Read the model definition and answer for the solid it produces. Units are mm, in the model's axes. A direction names the side the tool comes from. Give positions to 0.01 mm unless a question says otherwise; leave off trailing zeros. Loops run counter-clockwise (first coordinate to the right, second up) from the corner with the lowest first, then second, coordinate; pieces in that order, holes last.
(1) Find section D-D, the plane z = -4.75. Write down the section's boundary in (x, y).
(2) Straight lines are drawn through the part: probe 1 along Z at (x, y) = (9.75, 0); probe 2 along Y at (x, z) = (10.75, 0); probe 3 along Z at (x, y) = (13, 10.5). For each, find the intervals that lie inside material, in ascending order.
(3) Find section C-C, the plane z = 10.75. Write down the section's boundary in (x, y), then the cut area to 3 significant figures.
(4) Which of the six approach directions +Z, -Z, +X, -X, +Y, -Y give full straight-line access (tool end or side, diameter ignored) to faces 1 (the face through (6.9, -2.95, -10.79)), 2 (the face through (6.902, 10.082, 4.746)), 3 (the face through (6.902, 4.851, 8.384)), 4 (the face through (6.9, -11.14, 1.03))?
(5) Find section A-A, the plane z = 0. Write down the section's boundary in (x, y).
(6) Find section B-B, the plane y = -1.5. Write down the section's boundary in (x, z), then the cut area to 3 significant figures.
(7) Each of these flat-tipped pins is pushed along its axis until it touches: P1, Ø3, axis at x = 10, y = -9.5, coming from the -Z side; P2, Ø5, axis at x = 4.5, z = 4.5, coming from the -Y side; P3, Ø2, axis at x = 11.5, y = 6, coming from the +Z side. Where does it stop, or does it pass through?
(8) Determine the mould class of faces 5 (the face through (6.902, 6.425, -9.105)), 6 (the face through (6.9, 7.85, 7.91)), 7 (the face through (6.9, 2.95, 10.79)), 8 (the face through (14, 3, 0)) for opening direction Z: pulls with the +Z half, pulls with the -Z half, needs draft (parallel to the pull), parting line crosses it, or undercut.
```python
from build123d import *

# Parameters (mm, degrees)
BASPROSKE_W           = 14
BASPROSKE_H           = 12.5
TOOTHCUT_DEPTH        = 23.549944568
TEETHCUTS_COUNT       = 18
BORSKE_R              = 0.4
BORE_DEPTH            = 50.0000508
CORTAR_EXTRUIR1_REACH = 24.473


with BuildPart() as part:
    # BasProSke → Base-Revolve (revolve)
    with BuildSketch(Plane(origin=(0, 0, 0), x_dir=(1, 0, 0), z_dir=(0, 1, 0)), mode=Mode.PRIVATE) as base_revolve_sk:
        with Locations((7, 6.25)):
            Rectangle(BASPROSKE_W, BASPROSKE_H)
    revolve(base_revolve_sk.sketch.rotate(Axis((-10, 0, 0), (1, 0, 0)), 180), axis=Axis((-10, 0, 0), (1, 0, 0)))

    # TooCutSke → ToothCut (cut, through all)
    with BuildSketch(Plane(origin=(0, 0, 0), x_dir=(0, 0, -1), z_dir=(1, 0, 0))):
        with BuildLine():
            ThreePointArc((0.634554124, 9.665693111), (0, 9.6865), (-0.634554124, 9.665693111))
            ThreePointArc((-0.634554124, 9.665693111), (-1.026818848, 11.131124412), (-1.883745888, 12.38293772))
            ThreePointArc((-1.883745888, 12.38293772), (0, 12.5254), (1.883745888, 12.38293772))
            ThreePointArc((1.883745888, 12.38293772), (1.026818848, 11.131124412), (0.634554124, 9.665693111))
        make_face()
    toothcut = extrude(amount=TOOTHCUT_DEPTH, mode=Mode.SUBTRACT)

    # TeethCuts: ToothCut ×18 about axis
    teethcuts_axis = Axis((0, 0, 0), (1, 0, 0))
    for i in range(1, TEETHCUTS_COUNT):
        add(toothcut.rotate(teethcuts_axis, i * 360 / TEETHCUTS_COUNT), mode=Mode.SUBTRACT)

    # BorSke → Bore (cut, symmetric)
    with BuildSketch(Plane(origin=(0, 0, 0), x_dir=(0, 0, -1), z_dir=(1, 0, 0))):
        with Locations(Location((0, 0, 0), (0, 0, 180))):
            Circle(BORSKE_R)
    extrude(amount=BORE_DEPTH, both=True, mode=Mode.SUBTRACT)

    # Croquis1 → Cortar-Extruir1 (cut, up to next)
    with BuildSketch(Plane(origin=(14, 0, 0), x_dir=(0, 0, -1), z_dir=(1, 0, 0)), mode=Mode.PRIVATE) as cortar_extruir1_sk1:
        with BuildLine():
            Line((1.631716887, 1.4), (-1.631716887, 1.4))
            ThreePointArc((-1.631716887, 1.4), (-0.746427723, -2.016270233), (2.15, 0))
            ThreePointArc((2.15, 0), (2.016270233, 0.746427723), (1.631716887, 1.4))
        make_face()
    cortar_extruir1_tool1 = extrude(cortar_extruir1_sk1.sketch, amount=-CORTAR_EXTRUIR1_REACH, mode=Mode.PRIVATE) & part.part
    add(cortar_extruir1_tool1.solids().sort_by_distance((14, -0.225862, 0))[0], mode=Mode.SUBTRACT)


solid = part.part
```
Entries:
1. outline: (0, -10.09) - (14, -10.09) - (14, 10.09) - (0, 10.09) - close
2. probe 1: z = -12.5 to -2.15, 2.15 to 12.5
2. probe 2: y = -9.69 to -2.15, 1.4 to 9.69
2. probe 3: z = -6.53 to -5.21, -2.86 to -0.79, 0.79 to 2.86, 5.21 to 6.53
3. outline: (0, -4.69) - (14, -4.69) - (14, -2.92) - (0, -2.92) - close; (0, -1.01) - (14, -1.01) - (14, 1.01) - (0, 1.01) - close; (0, 2.92) - (14, 2.92) - (14, 4.69) - (0, 4.69) - close
3. area: 77.7 mm2
4. face 1: -Z, +X, -X
4. face 2: +X, -X, +Y
4. face 3: +X, -X
4. face 4: +X, -X, -Y
5. outline: (0, -9.69) - (14, -9.69) - (14, -2.15) - (0, -2.15) - close; (0, 1.4) - (14, 1.4) - (14, 9.69) - (0, 9.69) - close
6. outline: (0, -9.57) - (14, -9.57) - (14, -1.54) - (0, -1.54) - close; (0, 1.54) - (14, 1.54) - (14, 9.57) - (0, 9.57) - close
6. area: 225 mm2
7. P1: stops at z = -9.6
7. P2: stops at y = -12.34
7. P3: stops at z = 9.46
8. face 5: pulls with the -Z half
8. face 6: undercut
8. face 7: pulls with the +Z half
8. face 8: needs draft
